Read the model definition and answer for the solid it produces. Units are mm, in the model's axes. A direction names the side the tool comes from. Coordinates: 2 decimals unless noted, no trailing zeros. Write each loop counter-clockwise with the first axis right and the second up, starting at its lowest first coordinate (ties: lowest second). Pieces come first, ordered by that corner, then holes. Notation, with made-up numbers: (66.25, 13.5) -> (92.25, 13.5) arc R18 ccw to (92.25, 20.5) -> close; hole circle Ø1 at (-2, 6). An arc over 180 degrees is marked (long way). One line per item, written item: value. Start each with the question number.
1. For faces 5 (the flat face through (-2, 9.85, 5)), 6 (the cylindrical face through (-10.694, 11.497, -2.375)), 7 (the flat face through (-2, 13.19, 5)), determine the directions among +Z, -Z, +X, -X, +Y, -Y from which every point of the face is accessible in a straight line to the end or side of a thin tool.
2. Given P1, Ø6.5, axis at x = 0, z = -5.5, coming from the +Y side; P2, Ø5.5, axis at x = 8.1, z = 0.02, coming from the -Y side; P3, Ø7, axis at x = 0, z = 0, coming from the -Y side; P4, Ø1.5, axis at x = -2.5, y = 5, coming from the -Z side, each flat-ended and moving along its own axis, determine where each tip first touches the part or whether it passes through.
3. Find section A-A, the plane x = 8.1. Write down the section's boundary in (y, z), and give its area (3 significant figures).
4. Find section D-D, the plane x = 0. Write down the section's boundary in (y, z) (3 decimals).
5. Find section B-B, the plane z = -6.75. Write down the section's boundary in (x, y), and give its area (3 significant figures).
6. Find section C-C, the plane y = 12.5. Write down the section's boundary in (x, z) (3 decimals).
7. For a pull along Z with two mould halves and no side action, classify faces 1 (the cylindrical face through (1.52, 14.082, 4.826)), 2 (the cylindrical face through (-9.71, 11.5, -0.33)), 3 (the flat face through (2, 0, 4)), 4 (the cylindrical face through (0.496, 11.497, -6.502)) as pulls with the +Z half, pulls with the -Z half, needs draft (parallel to the pull), parting line crosses it, or undercut.
8. Consider line 1 along X through (y, z) = (5.75, 0); line 2 along Z through (x, y) = (1, 11.5); line 3 along Y through (x, z) = (-6, -2). Determine where each line is inside the solid, lowest interval first.
```python
from build123d import *

# Parameters (mm, degrees)
SKETCH_1_R      = 5.06
SKETCH_1_R_2    = 4
EXTRUDE_1_DEPTH = 15
EXTRUDE_START   = 9.85
SKETCH_1_3_R    = 10.955
SKETCH_1_3_R_2  = 1.65
SKETCH_1_3_R_3  = 5.06
EXTRUDE_2_DEPTH = 3.34


with BuildPart() as part:
    # Sketch 1 → Extrude 1 (new body)
    with BuildSketch(Plane(origin=(0, 0, 0), x_dir=(1, 0, 0), z_dir=(0, 1, 0))):
        with Locations(Location((0, 0, 0), (0, 0, 270))):
            Circle(SKETCH_1_R)
        with Locations(Location((0, 0, 0), (0, 0, 270))):
            Circle(SKETCH_1_R_2, mode=Mode.SUBTRACT)
    extrude(amount=EXTRUDE_1_DEPTH)

    # Sketch 1_3 → Extrude 2 (add)
    with BuildSketch(Plane(origin=(0, 0, 0), x_dir=(1, 0, 0), z_dir=(0, 1, 0)).offset(EXTRUDE_START)):
        with Locations(Location((0, 0, 0), (0, 0, 270))):
            Circle(SKETCH_1_3_R)
        with Locations(Location((-8.1, -0.024689505, 0), (0, 0, 270))):
            Circle(SKETCH_1_3_R_2, mode=Mode.SUBTRACT)
        with Locations(Location((0, -8.124689505, 0), (0, 0, 270))):
            Circle(SKETCH_1_3_R_2, mode=Mode.SUBTRACT)
        with Locations(Location((8.1, -0.024689505, 0), (0, 0, 270))):
            Circle(SKETCH_1_3_R_2, mode=Mode.SUBTRACT)
        with Locations(Location((0, 8.075310495, 0), (0, 0, 270))):
            Circle(SKETCH_1_3_R_2, mode=Mode.SUBTRACT)
        with Locations(Location((0, 0, 0), (0, 0, 270))):
            Circle(SKETCH_1_3_R_3, mode=Mode.SUBTRACT)
    extrude(amount=EXTRUDE_2_DEPTH)


solid = part.part
```
Answer block:
1. face 5: -Y
1. face 6: +Y, -Y
1. face 7: +Y
2. P1: stops at y = 15
2. P2: stops at y = 9.85
2. P3: passes through
2. P4: stops at z = -4.75
3. outline: (9.85, -7.38) -> (13.19, -7.38) -> (13.19, -1.63) -> (9.85, -1.63) -> close; (9.85, 1.67) -> (13.19, 1.67) -> (13.19, 7.38) -> (9.85, 7.38) -> close
3. area: 38.2 mm2
4. outline: (0, -5.06) -> (9.85, -5.06) -> (9.85, -6.425) -> (13.19, -6.425) -> (13.19, -5.06) -> (15, -5.06) -> (15, -4) -> (0, -4) -> close; (0, 4) -> (15, 4) -> (15, 5.06) -> (13.19, 5.06) -> (13.19, 6.475) -> (9.85, 6.475) -> (9.85, 5.06) -> (0, 5.06) -> close; (9.85, -10.955) -> (13.19, -10.955) -> (13.19, -9.725) -> (9.85, -9.725) -> close; (9.85, 9.775) -> (13.19, 9.775) -> (13.19, 10.955) -> (9.85, 10.955) -> close
5. outline: (-8.63, 9.85) -> (-0.98, 9.85) -> (-0.98, 13.19) -> (-8.63, 13.19) -> close; (0.98, 9.85) -> (8.63, 9.85) -> (8.63, 13.19) -> (0.98, 13.19) -> close
5. area: 51.1 mm2
6. outline: circle Ø21.91 at (0, 0); hole circle Ø3.3 at (-8.1, 0.025); hole circle Ø8 at (0, 0); hole circle Ø3.3 at (0, -8.075); hole circle Ø3.3 at (0, 8.125); hole circle Ø3.3 at (8.1, 0.025)
7. face 1: parting line crosses it
7. face 2: undercut
7. face 3: needs draft
7. face 4: undercut
8. line 1: x = -5.06 to -4, 4 to 5.06
8. line 2: z = -10.91 to -9.39, -6.76 to -3.87, 3.87 to 6.81, 9.44 to 10.91
8. line 3: y = 9.85 to 13.19
